Autodesk Inventor part; units mm, degrees
ref_plane "Work Plane1" through (0, 23, 0) normal (0, 1, 0) x (1, 0, 0)
ref_plane "YZ Plane" through (0, 0, 0) normal (1, 0, 0) x (0, 1, 0)
ref_plane "XZ Plane" through (0, 0, 0) normal (0, 1, 0) x (-1, 0, 0)
sketch "Sketch1" plane through (0, 0, 0) normal (0, 1, 0) x (-1, 0, 0)
  circle A0 centre (0, 0) radius 19.5
  circle A1 centre (0, 0) radius 20.5
  dimension "d0" = 39
  dimension "d1" = 41
extrude "Extrusion1" add sketch "Sketch1" along normal blind 16
thread "Thread1"
sketch "Sketch2" plane through (0, 16, 0) normal (0, 1, 0) x (1, 0, 0)
  circle A0 centre (0, 0) radius 20.5
  circle A1 centre (0, 0) radius 20.5
extrude "Extrusion2" add sketch "Sketch2" along normal blind 2
sketch "Sketch3" plane through (0, 18, 0) normal (0, 1, 0) x (1, 0, 0)
  circle A0 centre (0, 0) radius 2.5
  dimension "d8" = 5
extrude "Extrusion3" cut sketch "Sketch3" against normal blind 2
sketch "Sketch4" plane through (0, 18, 0) normal (0, 1, 0) x (1, 0, 0)
  circle A0 centre (0, 15) radius 4.5
  point P0 (0, 0)
  dimension "d13" = 9
  dimension "d14" = 15
ref_plane "Work Plane1" through (0, 23, 0) normal (0, 1, 0) x (1, 0, 0)
sketch "Sketch5" plane through (0, 23, 0) normal (0, 1, 0) x (1, 0, 0)
  circle A0 centre (0, 15) radius 3.5
  point P0 (0, 0)
  dimension "d16" = 7
loft "Loft1" add profiles "Sketch4", "Sketch5"
pattern_linear "Rectangular Pattern2" count 3 spacing 5 along (0, 1, 0) of "Loft1"
sketch "Sketch9" plane through (0, 33, -15) normal (0, 1, 0) x (1, 0, 0)
  circle A0 centre (0, 0) radius 3
  circle A1 centre (0, 0) radius 3.5
  point P0 (0, -15)
  dimension "d33" = 6
extrude "Extrusion5" cut sketch "Sketch9" against normal through all contours A0
properties part number "Cap" material "PPS Plastic"
Design review of the part built by this model. Coordinates are the model's own, in mm. A direction names the side the tool comes from. Round coordinates to 2 decimals unless told otherwise and drop trailing zeros. Write each loop counter-clockwise with the first axis right and the second up, starting at its lowest first coordinate (ties: lowest second). Pieces come first, ordered by that corner, then holes. Notation, with made-up numbers: (-24, 51.5) -> (27, 51.5) arc R10 cw to (27, 65.5) -> close; hole circle Ø7 at (45.25, 81). An arc over 180 degrees is marked (long way). One line per item, written item: value. Start each with the question number.
Q1. Insertion check: P1, Ø12, axis at y = 17, z = -11, coming from the +X side; P2, Ø6, axis at x = 0, z = 0, coming from the +Y side; P3, Ø4, axis at x = 3.5, y = 9.5, coming from the -Z side; P4, Ø10, axis at x = 1, z = -15, coming from the -Y side. Each pin has a flat end and moves straight along its axis. Give the tip position at first contact, or say it passes through.
Q2. Add section D-D (y = 31). Give the boundary of the cut face in (x, z), then the cut area to 3 significant figures.
Q3. Tool access review of faces 4 (the face through (0, 16, 4)), 5 (the face through (0, 23, -11)), 6 (the face through (-11, 0, -17)): name each direction out of +Z, -Z, +X, -X, +Y, -Y from which nothing blocks a thin tool from reaching the whole face with its end or side.
Q4. The part is to be moulded in two halves that separate along Z. For faces 1 (the face through (-0.507, 31.021, -11.137)), 2 (the face through (-0.54, 17.01, 2.44)), 3 (the face through (0, 18, 4)), say which applies: pulls with the +Z half, pulls with the -Z half, needs draft (parallel to the pull), parting line crosses it, or undercut.
Q5. Add section C-C (z = -8.5). Give the boundary of the cut face in (x, y).
Q6. To check wall thickness, follow probe 1 along Z at (x, y) = (0, 8.75); probe 2 along Y at (x, z) = (-15.5, 3); probe 3 along X at (y, z) = (6.5, -6). State the ranges of each line that lie inside material, in increasing order.
Q7. Add section B-B (y = 10). Give the boundary of the cut face in (x, z).
Response:
1. P1: stops at x = 19.88
1. P2: stops at y = 18
1. P3: stops at z = -20.45
1. P4: stops at y = 0
2. outline: circle Ø7.8 at (0, -15); hole circle Ø6 at (0, -15)
2. area: 19.5 mm^2
3. face 4: -Y
3. face 5: none
3. face 6: +Z, -Z, +X, -X, -Y
4. face 1: parting line crosses it
4. face 2: undercut
4. face 3: needs draft
5. outline: (-18.65, 0) -> (-17.55, 0) -> (-17.55, 16) -> (17.55, 16) -> (17.55, 0) -> (18.65, 0) -> (18.65, 18) -> (-18.65, 18) -> close
6. probe 1: z = -20.5 to -19.5, 19.5 to 20.5
6. probe 2: y = 16 to 18
6. probe 3: x = -19.6 to -18.55, 18.55 to 19.6
7. outline: circle Ø41 at (0, 0); hole circle Ø39 at (0, 0)
